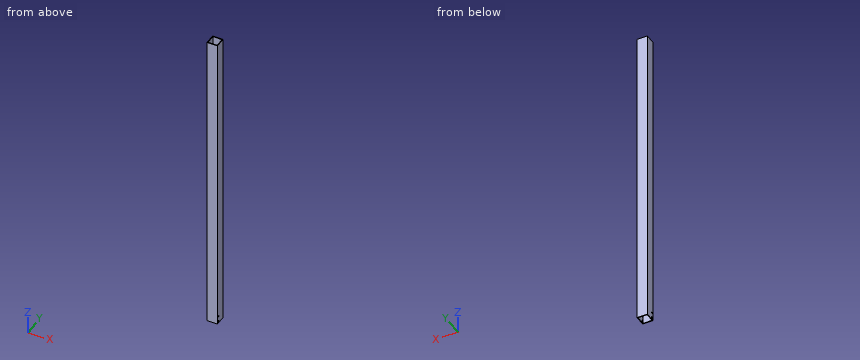
```python
from build123d import *

# Parameters (mm, degrees)
F0_W     = 25.4
F0_H     = 25.4
F0_W_2   = 22.225
F0_H_2   = 22.225
F1_DEPTH = 762
F2_R     = 1.8288
F3_DEPTH = 25.4


with BuildPart() as f1:
    # F0 (on Top) → F1 (new body)
    with BuildSketch(Plane.XY):
        Rectangle(F0_W, F0_H)
        Rectangle(F0_W_2, F0_H_2, mode=Mode.SUBTRACT)
    extrude(amount=F1_DEPTH)

    # F2 (on face) → F3 (cut, through all)
    with BuildSketch(Plane.YZ.offset(12.7)):
        with Locations((-7.9375, 4.7625)):
            Circle(F2_R)
        with Locations((-7.9375, 17.4625)):
            Circle(F2_R)
    extrude(amount=-F3_DEPTH, mode=Mode.SUBTRACT)


solid = f1.part
```
Check sheet for the modelled part. Datum: model origin and axes. Units: mm. Round coordinates to 2 decimals unless told otherwise and drop trailing zeros. Loops run counter-clockwise (first coordinate to the right, second up) from the corner with the lowest first, then second, coordinate; pieces in that order, holes last. Notation, with made-up numbers: (-24.5, -8.5) - (-4.5, -8.5) arc R6 ccw to (-4.5, -2.5) - close; hole circle Ø9 at (66.5, 81). An arc over 180 degrees is marked (long way). Answer as a JSON object with one key per item and string values. Group by question number.
Q1. Sectioned sample at A-A, the plane x = 2.5. Enter the section's corners in (y, z).
Q2. Scan line: line 1 along Y through (x, z) = (0.5, 714.5). Record every from-to range of solid material in increasing order. Write a range as [from, to].
Q3. Gauge pin test, flat end, axial feed: P1, Ø3.5, axis at y = -7.94, z = 4.76, coming from the -X side. Record the tip position at first contact, or that the pin passes through.
Q4. Sectioned sample at B-B, the plane z = 364. Enter the section's corners in (x, y), plus the area to 3 significant figures.
Solution:
{
 "1": {"outline": "(-12.7, 0) - (-11.11, 0) - (-11.11, 762) - (-12.7, 762) - close; (11.11, 0) - (12.7, 0) - (12.7, 762) - (11.11, 762) - close"},
 "2": {"line 1": "y = [-12.7, -11.11], [11.11, 12.7]"},
 "3": {"P1": "passes through"},
 "4": {"outline": "(-12.7, -12.7) - (12.7, -12.7) - (12.7, 12.7) - (-12.7, 12.7) - close; hole (-11.11, -11.11) - (11.11, -11.11) - (11.11, 11.11) - (-11.11, 11.11) - close", "area": "151 mm²"}
}
